Autodesk Inventor part; units mm, degrees
ref_plane "Work Plane1" through (1.525, 0, 0) normal (0, 0, 1) x (1, 0, 0)
ref_plane "YZ Plane" through (0, 0, 0) normal (1, 0, 0) x (0, 1, 0)
ref_plane "XZ Plane" through (0, 0, 0) normal (0, 1, 0) x (-1, 0, 0)
sketch "Sketch1" plane through (0, 0, 0) normal (0, 0, 1) x (1, 0, 0)
  line L0 (0, 7.1374) -> (0, 4.7625)
  line L1 (19.05, 4.7625) -> (44.45, 4.7625)
  line L2 (44.45, 4.7625) -> (44.45, 0)
  line L3 (44.45, 0) -> (-0.6351, 0)
  line L4 (-9.6521, 0) -> (53.467, 0)
  line L5 (-0.6351, 0) -> (-0.6351, 7.1374)
  line L6 (-0.6351, 7.1374) -> (0, 7.1374)
  line L7 (19.05, 4.7625) -> (7.9247, 4.7625)
  line L8 (7.9247, 4.7625) -> (0, 4.7625)
  line L9 (0, -1.4275) -> (0, 8.5649)
  dimension "d0" = 44.45
  dimension "d1" = 25.4
  dimension "d2" = 9.525
  dimension "d9" = 0.6351
  dimension "d10" = 14.2748
  dimension "d13" = 11.1253
  dimension "d14" = 9.525
revolve "Body" add sketch "Sketch1" angle 360 about axis through (44.45, 0, 0) along (-1, 0, 0)
sketch "Sketch2" plane through (-0.6351, 0, 0) normal (-1, 0, 0) x (0, 0, 1)
  line L0 (0, 8.2416) -> (7.1374, 4.1208)
  line L1 (7.1374, 4.1208) -> (7.1374, -4.1208)
  line L2 (7.1374, -4.1208) -> (0, -8.2416)
  line L3 (0, -8.2416) -> (-7.1374, -4.1208)
  line L4 (-7.1374, -4.1208) -> (-7.1374, 4.1208)
  line L5 (-7.1374, 4.1208) -> (0, 8.2416)
  point P0 (0, 0)
  point P1 (0, 0)
  dimension "d11" = 14.2748
extrude "Head" add sketch "Sketch2" along normal blind 5.5372
sketch "Sketch4" plane through (0, 0, 0) normal (0, 0, 1) x (1, 0, 0)
  line L0 (-6.1723, 7.1374) -> (-6.1723, 8.2416)
  line L1 (-6.1723, 8.2416) -> (-5.5348, 8.2416)
  line L2 (-5.5348, 8.2416) -> (-6.1723, 7.1374)
  line L3 (-7.2797, 0) -> (0.4723, 0)
  line L4 (-0.6351, 8.2416) -> (-6.1723, 8.2416)
  line L5 (-6.1723, 4.1208) -> (-6.1723, 8.2416)
  dimension "d5" = 30
  dimension "d19" = 14.2748
revolve "Chamfer1" cut sketch "Sketch4" angle 360 about axis through (-10, 0, 0) along (1, 0, 0)
thread "Thread"
chamfer "Chamfer2" distance 0.9738 distance2 0.9739 1 edges at (44.45, -4.7625, 0) measured on face at (44.45, -1.2549, 0.1261)
ref_plane "Work Plane1" through (1.525, 0, 0) normal (0, 0, 1) x (1, 0, 0)
equation "\"d0\" = NLG"
equation "\"d1\" = GEL"
equation "\"d2\" = GD"
equation "\"d10\" = SD2"
equation "\"d14\" = BDM"
equation "\"d11\" = SW"
equation "\"d3\" = KOH - SD"
equation "\"d5\" = ANG1"
equation "\"d19\" = SW0"
equation "\"d15\" = GEL"
equation "\"d6\" = -0.5 * SPD + 0.5 * GD"
equation "\"NLG\" = 44.45"
equation "\"GD\" = 9.525"
equation "\"BDM\" = 9.525"
equation "\"KOH\" = 6.1722"
equation "\"GEL\" = 25.4"
equation "\"SW\" = 14.2748"
equation "\"SW0\" = SW"
equation "\"SPD\" = GD1"
equation "\"SD2\" = SW"
equation "\"SD\" = 0.635"
equation "\"ANG1\" = 30deg"
equation "\"GAL\" = 11.1252"
equation "\"GUL\" = 0.97384"
equation "\"RR\" = 0.381"
equation "\"WFT\" = SD"
equation "\"GD1\" = 7.57733"
equation "\"THREADDIA\" = 9.525"
equation "\"SDH\" = SW"
equation "\"SDHG\" = 7.9248"
equation "\"TOA\" = 30deg"
equation "\"FAWI\" = 45deg"
equation "\"NND\" = 9.525"
equation "\"E0\" = 16.48739"
properties part number "AS 2465 - 3/8 x 1 3/4  UNC" material "Steel, Mild"
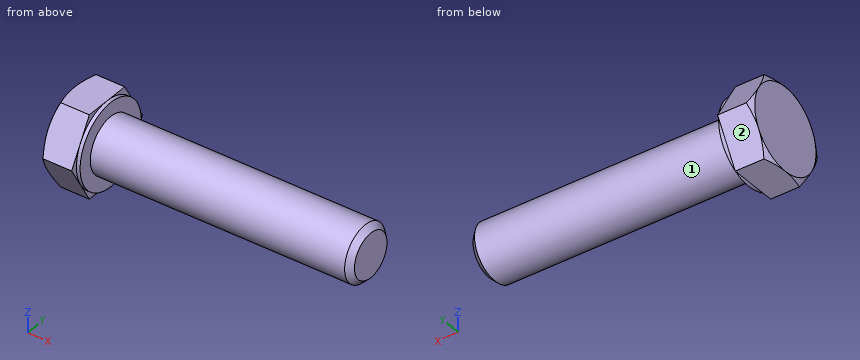
Here's how the part is built. I have some questions about the finished solid (model axes, mm). Face numbers are marked on the shaded views. A direction names the side the tool comes from. Coordinates: 2 decimals unless noted, no trailing zeros. Write each loop counter-clockwise with the first axis right and the second up, starting at its lowest first coordinate (ties: lowest second). Pieces come first, ordered by that corner, then holes. Notation, with made-up numbers: (-23.75, 19.25) - (8.25, 19.25) arc R21 cw to (8.25, 37.25) - close; hole circle Ø5 at (43, -20). An arc over 180 degrees is marked (long way). Use one line per item in the form item = value.
1) On a 3-axis mill with a long thin cutter (end or side, diameter ignored), from which of +Z, -Z, +X, -X, +Y, -Y can I reach the whole of each face in a straight line? I mean the marked faces 1 and 2. Say none if no direction works.
Solved:
face_1 = +X
face_2 = -Z, +X, -X, +Y
2) I need wall thicknesses on line 1 (X direction, y = -6, z = 2.5); line 2 (Z direction, x = 17, y = 0); line 3 (Y direction, x = 36, z = -1.5). Which ranges of each line are inside material? Lowest first, please.
Solved:
line_1 = -6.17 to 0
line_2 = -4.76 to 4.76
line_3 = -4.52 to 4.52
3) I'm going to push flat-ended pins straight in: P1, Ø3, axis at x = 37, y = -2, coming from the -Z side; P2, Ø4, axis at x = 34, z = -1.5, coming from the -Y side; P3, Ø1, axis at x = 13, y = 0, coming from the +Z side. Where does each tip first touch, or does it pass through?
Solved:
P1 = -4.74
P2 = -4.76
P3 = 4.76
4) Suppose I cut it at A-A, the plane x = 21. Write out the boundary of the cut face in (y, z) (1 decimal).
Solved:
outline = circle Ø9.5 at (0, 0)
